Design review of the part shown in the three views and the two pictorial views. Dimensions are in mm from the part's minimum x, y and z. A direction names the side the tool comes from. Round coordinates to 2 decimals unless told otherwise and drop trailing zeros. Loops run counter-clockwise (first coordinate to the right, second up) from the corner with the lowest first, then second, coordinate; pieces in that order, holes last.
1) Take a section at D-D (x = 23). State the section outline as (y, z) points, then the cut area to 3 significant figures.
2) Wall thickness on L1, parallel to X at y = 8, z = 36.5; L2, parallel to Z at x = 17.5, y = 3.5; L3, parallel to Y at x = 41.5, z = 39: over which ranges is each line inside the solid? List them lowest first.
3) Take a section at A-A (x = 48). State the section outline as (y, z) points, then the cut area to 3 significant figures.
4) Mouldability with a two-part tool opening along Z and no side actions: class the marked faces 3, 4 and 5 as pulls with the +Z half, pulls with the -Z half, needs draft (parallel to the pull), parting line crosses it, or undercut.
5) Take a section at C-C (z = 9). State the section outline as (x, y) points, then the cut area to 3 significant figures.
6) Take a section at B-B (y = 9.5). State the section outline as (x, z) points.
7) Tool access review of the marked faces 1 and 2: name each direction out of +Z, -Z, +X, -X, +Y, -Y from which nothing blocks a thin tool from reaching the whole face with its end or side.
8) Insertion check: pin 1 (12 mm diameter, centred on x = 59, z = 21, fed in from +Y); pin 2 (1.6 mm diameter, centred on y = 10, z = 66.5, fed in from +X); pin 3 (2 mm diameter, centred on y = 9.5, z = 1, fed in from +X). Each pin has a flat end and moves straight along its axis. Give the tip position at first contact, or say it passes through.
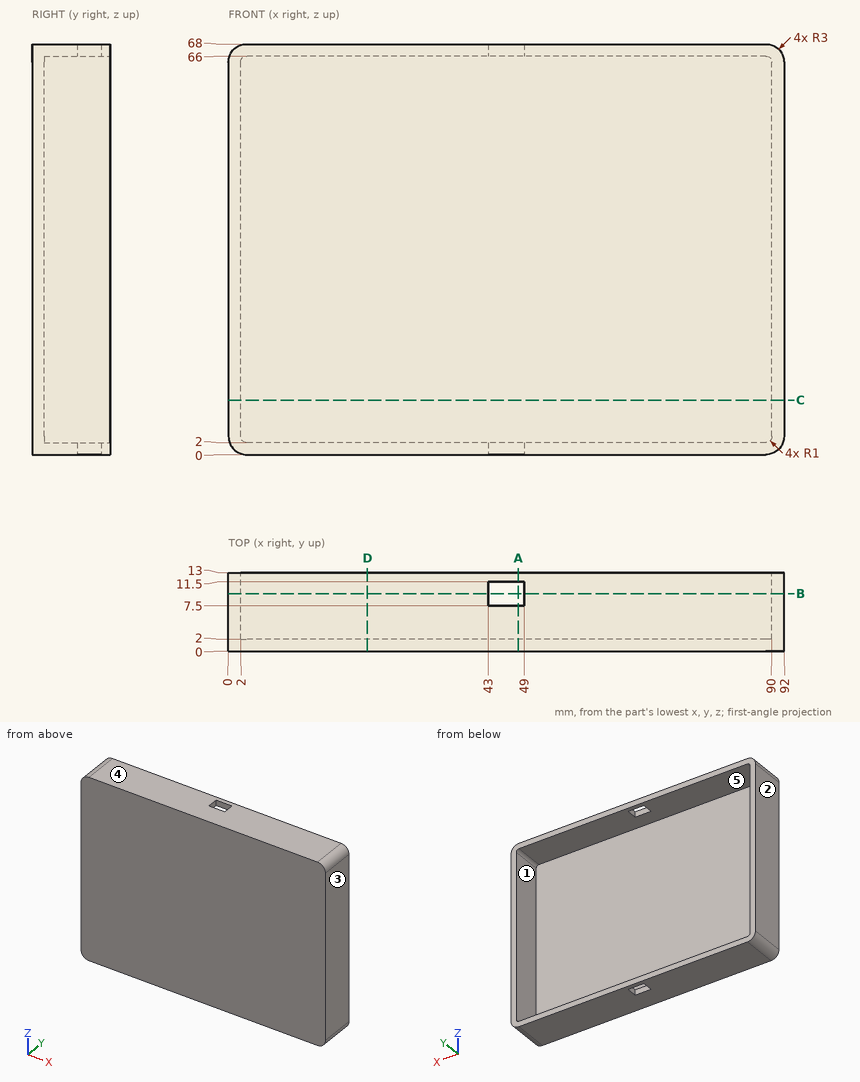
Response:
1. outline: (0, 0) - (13, 0) - (13, 2) - (2, 2) - (2, 66) - (13, 66) - (13, 68) - (0, 68) - close
1. area: 180 mm2
2. L1: x = 0 to 2, 90 to 92
2. L2: z = 0 to 2, 66 to 68
2. L3: y = 0 to 2
3. outline: (0, 0) - (7.5, 0) - (7.5, 2) - (2, 2) - (2, 66) - (7.5, 66) - (7.5, 68) - (0, 68) - close; (11.5, 0) - (13, 0) - (13, 2) - (11.5, 2) - close; (11.5, 66) - (13, 66) - (13, 68) - (11.5, 68) - close
3. area: 164 mm2
4. face 3: needs draft
4. face 4: pulls with the +Z half
4. face 5: undercut
5. outline: (0, 0) - (92, 0) - (92, 13) - (90, 13) - (90, 2) - (2, 2) - (2, 13) - (0, 13) - close
5. area: 228 mm2
6. outline: (0, 3) arc R3 ccw to (3, 0) - (43, 0) - (43, 2) - (3, 2) arc R1 cw to (2, 3) - (2, 65) arc R1 cw to (3, 66) - (43, 66) - (43, 68) - (3, 68) arc R3 ccw to (0, 65) - close; (49, 0) - (89, 0) arc R3 ccw to (92, 3) - (92, 65) arc R3 ccw to (89, 68) - (49, 68) - (49, 66) - (89, 66) arc R1 cw to (90, 65) - (90, 3) arc R1 cw to (89, 2) - (49, 2) - close
7. face 1: +Y
7. face 2: +Z, -Z, -X, +Y, -Y
8. pin 1: stops at y = 2
8. pin 2: stops at x = 91.92
8. pin 3: stops at x = 91.83
